Build history of the part. All positions in model axes, mm. A direction names the side the tool comes from. Give positions to 0.01 mm unless a question says otherwise; leave off trailing zeros. Order: outer loops, then holes, each group sorted by start corner. A loop starts at its lowest first (then second) coordinate and runs counter-clockwise, first axis right, second up. Notation, with made-up numbers: (61.5, 38) - (111.5, 38) arc R19 cw to (111.5, 75) - close; hole circle Ø10 at (10.5, 18.5). An arc over 180 degrees is marked (long way). Answer in a Markdown table with one row per item.
Autodesk Fusion 360 part; units mm, degrees
sketch "Sketch1" plane through (0, 0, 0) normal (0, 0, 1) x (1, 0, 0)
  line L0 (15, -15) -> (-15, -15)
  line L1 (-15, -15) -> (-15, 15)
  line L2 (-15, 15) -> (15, 15)
  line L3 (15, 15) -> (15, -15)
  line L4 (15, -15) -> (-15, 15) construction
  line L5 (-15, -15) -> (15, 15) construction
  dimension "d1" = 30
  dimension "d2" = 30
extrude "Extrude1" add sketch "Sketch1" along normal blind 4
sketch "Sketch2" plane through (0, 0, 0) normal (0, 0, -1) x (1, 0, 0)
  line L0 (-15, -15) -> (15, -15)
  line L1 (15, -15) -> (15, 15)
  line L2 (15, 15) -> (-15, 15)
  line L3 (-15, 15) -> (-15, -15)
  line L4 (-15, 15) -> (-13, 15)
  line L5 (-13, 13) -> (-15, 13)
  line L6 (-13, 15) -> (-13, 13)
extrude "Extrude2" add sketch "Sketch2" along normal blind 30 contours L2 L3 L4 L5 L6
mirror "Mirror1" about plane through (0, 0, 0) normal (1, 0, 0) of "Extrude2"
mirror "Mirror2" about plane through (0, 0, 0) normal (0, 1, 0) of "Extrude2", "Mirror1"
1. Two-plate mould, pull along Y, no slides. Class faces 1 (the face through (0, -15, 1)), 2 (the face through (14, -13, -15)), 3 (the face through (-14, 13, -15)), 4 (the face through (-14, -14, -30)): +Y half, -Y half, draft (parallel to the pull), parting line (faces both ways), or undercut.
Check result:
| item | result |
|---|---|
| face 1 | -Y half |
| face 2 | undercut |
| face 3 | undercut |
| face 4 | draft |
2. Probe line 1 (Z direction, x = 5.5, y = -9). List the from-to ranges inside material, lowest first.
Check result:
| item | result |
|---|---|
| line 1 | z = 0 to 4 |
3. Cut at B-B on y = 11.25. Write the cut outline in (x, z), and give its area (3 significant figures).
Check result:
| item | result |
|---|---|
| outline | (-15, 0) - (15, 0) - (15, 4) - (-15, 4) - close |
| area | 120 mm² |
4. Cut at A-A on z = -8.5. Write the cut outline in (x, y).
Check result:
| item | result |
|---|---|
| outline | (-15, -15) - (-13, -15) - (-13, -13) - (-15, -13) - close; (-15, 13) - (-13, 13) - (-13, 15) - (-15, 15) - close; (13, -15) - (15, -15) - (15, -13) - (13, -13) - close; (13, 13) - (15, 13) - (15, 15) - (13, 15) - close |
5. Drop flat-ended pins along their axis: P1, Ø12, axis at x = -5, z = -12, coming from the +Y side; P2, Ø15, axis at x = 0, y = 0.5, coming from the -Z side. Give the stop position or say it passes through.
Check result:
| item | result |
|---|---|
| P1 | passes through |
| P2 | stops at z = 0 |
6. Which spindle directions (+Z, -Z, +X, -X, +Y, -Y) get a long thin tool onto all of the face, cutting with end or side? Do faces 5 (the face through (-14, -13, -15)), 6 (the face through (13, -14, -15)), 7 (the face through (14, -14, -30)). Say none if no direction does.
Check result:
| item | result |
|---|---|
| face 5 | -Z, +X, -X |
| face 6 | -Z, +Y, -Y |
| face 7 | -Z, +X, -X, +Y, -Y |
